from build123d import *

# Parameters (mm, degrees)
BOSS_EXTRUDE1_DEPTH = 7
BOSS_EXTRUDE2_DEPTH = 2
CUT_EXTRUDE1_START  = 6.5
CUT_EXTRUDE1_DEPTH  = 31.789915603
FILLET1_R           = 2
SKETCH2_R           = 0.8
SCREW_HOLES_DEPTH   = 25.289915673
SKETCH4_R           = 1.25
SCREW_HEADS_DEPTH   = 3


with BuildPart() as part:
    # Sketch5 → Boss-Extrude1 (new body)
    with BuildSketch(Plane(origin=(0, 0, 0), x_dir=(1, 0, 0), z_dir=(0, 1, 0))):
        with BuildLine():
            Line((-10, -6.5), (10, -6.5))
            Line((10, -6.5), (10, 4.202041029))
            ThreePointArc((10, 4.202041029), (0, 0), (-10, 4.202041029))
            Line((-10, 4.202041029), (-10, -6.5))
        make_face()
    extrude(amount=-BOSS_EXTRUDE1_DEPTH)

    # Sketch6 → Boss-Extrude2 (add)
    with BuildSketch(Plane(origin=(0, 0, 0), x_dir=(1, 0, 0), z_dir=(0, 1, 0))):
        Polygon((-7, 14), (-7, 0), (7, 0), (7, 14), (4, 21), (0, 21), (-4, 21), align=None)
    extrude(amount=-BOSS_EXTRUDE2_DEPTH)

    # Sketch3 → Cut-Extrude1 (cut, through all)
    with BuildSketch(Plane.XY.offset(CUT_EXTRUDE1_START)):
        with BuildLine():
            Line((3, -7), (3, -5.5))
            ThreePointArc((3, -5.5), (2.560660172, -4.439339828), (1.5, -4))
            Line((1.5, -4), (-1.5, -4))
            ThreePointArc((-1.5, -4), (-2.560660172, -4.439339828), (-3, -5.5))
            Line((-3, -5.5), (-3, -7))
            Line((-3, -7), (0, -7))
            Line((0, -7), (3, -7))
        make_face()
    extrude(amount=-CUT_EXTRUDE1_DEPTH, mode=Mode.SUBTRACT)

    # Fillet1
    fillet1_edges = [part.edges().sort_by_distance(p)[0] for p in [
        (10, 0, 1.148979486),
        (-10, 0, 1.148979486),
        (7, 0, -7.937822174),
        (-7, 0, -7.937822174),
        (0, 0, -21),
        (-5.5, 0, -17.5),
        (5.5, 0, -17.5),
    ]]
    fillet(fillet1_edges, radius=FILLET1_R - 0.0001)  # a hair under: the kernel refuses the full size

    # Sketch2 → Screw Holes (cut, through all)
    with BuildSketch(Plane(origin=(0, 0, 0), x_dir=(1, 0, 0), z_dir=(0, 1, 0))):
        with Locations(Location((-8, -1.5, 0), (0, 0, 270))):
            Circle(SKETCH2_R)
        with Locations(Location((8, -1.5, 0), (0, 0, 270))):
            Circle(SKETCH2_R)
        with Locations(Location((8, -4.5, 0), (0, 0, 270))):
            Circle(SKETCH2_R)
        with Locations(Location((-8, -4.5, 0), (0, 0, 270))):
            Circle(SKETCH2_R)
    extrude(amount=-SCREW_HOLES_DEPTH, mode=Mode.SUBTRACT)

    # Sketch4 → Screw Heads (cut)
    with BuildSketch(Plane(origin=(0, 0, 0), x_dir=(1, 0, 0), z_dir=(0, 1, 0))):
        with Locations(Location((-8, -1.5, 0), (0, 0, 270))):
            Circle(SKETCH4_R)
        with Locations(Location((8, -1.5, 0), (0, 0, 270))):
            Circle(SKETCH4_R)
    extrude(amount=-SCREW_HEADS_DEPTH, mode=Mode.SUBTRACT)


solid = part.part
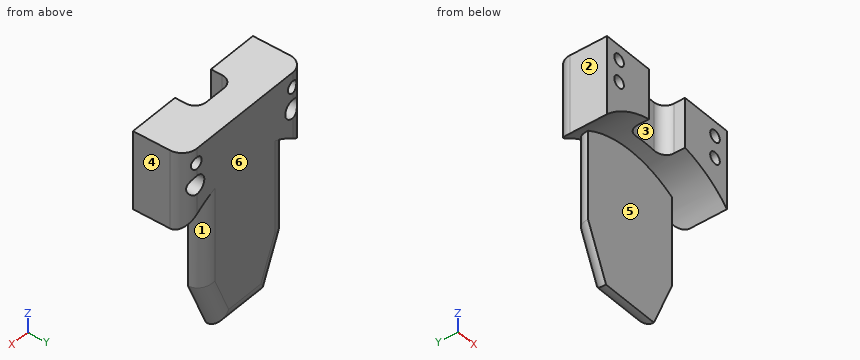
Can you work these out from the model? Positions are in its coordinate system, mm. Face numbers are marked on the shaded views. A direction names the side the tool comes from. Coordinates: 2 decimals unless noted, no trailing zeros. Loops run counter-clockwise (first coordinate to the right, second up) from the corner with the lowest first, then second, coordinate; pieces in that order, holes last. Notation, with made-up numbers: (8, 56.25) - (45, 56.25) arc R14 ccw to (45, 75.25) - close; hole circle Ø10 at (44, 35.5). An arc over 180 degrees is marked (long way). Answer as a JSON object with one key per item and string values. Group by question number.
Item 1: If we section it at A-A (z = 4.5): List the corners of the cut face in (x, y) for me.
Item 2: If we section it at B-B (y = -2.5): List the corners of the cut face in (x, z) for me.
Item 3: On a 3-axis mill with a long thin cutter (end or side, diameter ignored), from which of +Z, -Z, +X, -X, +Y, -Y can I reach the whole of each face in a straight line? I mean the marked faces 1, 2 and 3. Say none if no direction works.
Item 4: If we mould it in two halves opening along X, with no side actions, what happens to the marked faces 4, 5 and 6? For each: released by +X, released by -X, zero draft, split by the parting line, or undercut.
Item 5: For pin 1 (4 mm diameter, centred on x = 6.5, z = -2, fed in from -Y); pin 2 (4 mm diameter, centred on x = 0.5, z = -8, fed in from -Y); pin 3 (2 mm diameter, centred on x = 8, z = 1.5, fed in from +Y); pin 4 (2.5 mm diameter, centred on x = 0.5, z = 3, fed in from -Y), each with a flat end and sliding along its axis, tell me the tip position at first contact or that it passes through.
Item 6: If we section it at D-D (z = 1.5): List the corners of the cut face in (x, y) for me.
Item 7: If I drill on L1, parallel to X at y = -3.75, z = 4.5; L2, parallel to X at y = -5.5, z = 1.5; L3, parallel to Z at x = -8, y = -2.25, over which ranges is the centre line in solid material (lowest first)? Write a range as from..to.
Item 8: If we section it at C-C (x = -7.5): List the corners of the cut face in (y, z) for me, plus the area to 3 significant figures.
Returned:
{
 "1": {"outline": "(-10, -7) - (-8.8, -7) - (-8.8, -0.17) arc R2 ccw to (-10, -2) - close; (-7.2, -7) - (-3, -7) - (-3, -5.5) arc R1.5 cw to (-1.5, -4) - (1.5, -4) arc R1.5 cw to (3, -5.5) - (3, -7) - (7.2, -7) - (7.2, 0) - (-7.2, 0) - close; (8.8, -7) - (10, -7) - (10, -2) arc R2 ccw to (8.8, -0.17) - close"},
 "2": {"outline": "(-10, -4.2) arc R14 cw to (10, -4.2) - (10, 6.5) - (-10, 6.5) - close; hole circle Ø2.5 at (-8, 1.5); hole circle Ø1.6 at (-8, 4.5); hole circle Ø2.5 at (8, 1.5); hole circle Ø1.6 at (8, 4.5)"},
 "3": {"face 1": "-Z, +Y", "face 2": "+Z, -Z, -X, +Y, -Y", "face 3": "+Z, -Z, -Y"},
 "4": {"face 4": "released by +X", "face 5": "undercut", "face 6": "zero draft"},
 "5": {"pin 1": "stops at y = -7", "pin 2": "stops at y = -2", "pin 3": "stops at y = -3", "pin 4": "stops at y = -4.02"},
 "6": {"outline": "(-10, -7) - (-8.8, -7) - (-8.8, -3) - (-9.25, -3) - (-9.25, -0.44) arc R2 ccw to (-10, -2) - close; (-7.2, -7) - (-3, -7) - (-3, -5.5) arc R1.5 cw to (-1.5, -4) - (1.5, -4) arc R1.5 cw to (3, -5.5) - (3, -7) - (7.2, -7) - (7.2, -3) - (6.75, -3) - (6.75, 0) - (-6.75, 0) - (-6.75, -3) - (-7.2, -3) - close; (8.8, -7) - (10, -7) - (10, -2) arc R2 ccw to (9.25, -0.44) - (9.25, -3) - (8.8, -3) - close"},
 "7": {"L1": "x = -10..-8.8, -7.2..7.2, 8.8..10", "L2": "x = -10..-8.8, -7.2..-3, 3..7.2, 8.8..10", "L3": "z = -2.51..0.25, 2.75..3.7, 5.3..6.5"},
 "8": {"outline": "(-7, -2.18) - (0, -2.18) - (0, 0.35) - (-3, 0.35) - (-3, 0.88) - (-7, 0.88) - close; (-7, 2.12) - (-3, 2.12) - (-3, 2.65) - (0, 2.65) - (0, 3.88) - (-7, 3.88) - close; (-7, 5.12) - (0, 5.12) - (0, 6.5) - (-7, 6.5) - close", "area": "40.1 mm²"}
}
